```python
from build123d import *

# Parameters (mm, degrees)
SKETCH1_W                = 60
SKETCH1_H                = 60
BOSS_EXTRUDE1_DEPTH      = 41
M3_CLEARANCE_HOLE1_D     = 3.4
M3_CLEARANCE_HOLE1_DEPTH = 7
M3_CLEARANCE_HOLE1_TIP   = 1.021463052
SKETCH4_W                = 50
SKETCH4_H                = 50
BOSS_EXTRUDE2_DEPTH      = 28
SKETCH5_W                = 56
SKETCH5_H                = 56
BOSS_EXTRUDE3_DEPTH      = 18


with BuildPart() as part:
    # Sketch1 → Boss-Extrude1 (new body)
    with BuildSketch(Plane(origin=(0, 0, 0), x_dir=(1, 0, 0), z_dir=(0, 1, 0))):
        with Locations((30, 30)):
            Rectangle(SKETCH1_W, SKETCH1_H)
    extrude(amount=BOSS_EXTRUDE1_DEPTH)

    # M3 Clearance Hole1
    with Locations(Plane(origin=(0, 0, 0), x_dir=(-1, 0, 0), z_dir=(0, -1, 0))):
        with Locations((-3.5, 3.5), (-56.5, 3.5), (-56.5, 56.5), (-3.5, 56.5)):
            Hole(M3_CLEARANCE_HOLE1_D / 2, depth=M3_CLEARANCE_HOLE1_DEPTH)
            with Locations((0, 0, -(M3_CLEARANCE_HOLE1_DEPTH + M3_CLEARANCE_HOLE1_TIP / 2))):  # 118° drill point
                Cone(0, M3_CLEARANCE_HOLE1_D / 2, M3_CLEARANCE_HOLE1_TIP, mode=Mode.SUBTRACT)

    # Sketch4 → Boss-Extrude2 (add)
    with BuildSketch(Plane(origin=(0, 41, 0), x_dir=(1, 0, 0), z_dir=(0, 1, 0))):
        with Locations((30, 30)):
            Rectangle(SKETCH4_W, SKETCH4_H)
    extrude(amount=BOSS_EXTRUDE2_DEPTH)

    # Sketch5 → Boss-Extrude3 (add)
    with BuildSketch(Plane(origin=(0, 69, 0), x_dir=(1, 0, 0), z_dir=(0, 1, 0))):
        with Locations((30, 30)):
            Rectangle(SKETCH5_W, SKETCH5_H)
    extrude(amount=BOSS_EXTRUDE3_DEPTH)


solid = part.part
```
The listing builds one solid part. Answer for the finished solid, in the listing's coordinates (mm). A direction names the side the tool comes from. Coordinates: 2 decimals unless noted, no trailing zeros. Write each loop counter-clockwise with the first axis right and the second up, starting at its lowest first coordinate (ties: lowest second). Pieces come first, ordered by that corner, then holes. Notation, with made-up numbers: M 68.5,-23.5 L 83.5,-23.5 A4 cw 83.5,-16.5 Z; hole C 66,41 d9. An arc over 180 degrees is marked long. Use a Markdown table: item, result. Add a question column.
1. For a pull along Y with two mould halves and no side action, classify faces 1 (the flat face through (55, 55, -30)), 2 (the flat face through (30, 87, -30)), 3 (the flat face through (30, 20, -60)) as +Y half, -Y half, draft (parallel to the pull), parting line (faces both ways), or undercut.
2. Section B-B (z = -22) is taken. Give the vertices of the cut face in (x, y).
3. Section A-A (x = 10) is taken. Give the vertices of the cut face in (y, z), plus the area to 3 significant figures.
4. Given P1, Ø20, axis at x = 28, y = 81.5, coming from the +Z side; P2, Ø6, axis at x = 26.5, y = 65.5, coming from the +Z side; P3, Ø22.5, axis at y = 57, z = -25.5, coming from the +X side, each flat-ended and moving along its own axis, determine where each tip first touches the part or whether it passes through.
5. Section C-C (y = 56) is taken. Give the vertices of the cut face in (x, z).
6. Which of the six approach directions +Z, -Z, +X, -X, +Y, -Y give full straight-line access (tool end or side, diameter ignored) to faces 4 (the flat face through (30, 78, -2)), 5 (the flat face through (2, 78, -30)), 6 (the flat face through (56, 41, -30)), 7 (the cylindrical face through (54.8, 3.55, -3.57))?
7. Straight lines are drawn through the part: line 1 along X through (y, z) = (5, -56.5); line 2 along Z through (x, y) = (56.5, 5.5); line 3 along Y through (x, z) = (56, -14). For each, find the intervals that lie inside material, in ascending order. Write a range as [from, to].
Data:
| question | item | result |
|---|---|---|
| 1 | face 1 | undercut |
| 1 | face 2 | +Y half |
| 1 | face 3 | draft |
| 2 | outline | M 0,0 L 60,0 L 60,41 L 55,41 L 55,69 L 58,69 L 58,87 L 2,87 L 2,69 L 5,69 L 5,41 L 0,41 Z |
| 3 | outline | M 0,-60 L 41,-60 L 41,-55 L 69,-55 L 69,-58 L 87,-58 L 87,-2 L 69,-2 L 69,-5 L 41,-5 L 41,0 L 0,0 Z |
| 3 | area | 4,870 mm2 |
| 4 | P1 | stops at z = -2 |
| 4 | P2 | stops at z = -5 |
| 4 | P3 | stops at x = 55 |
| 5 | outline | M 5,-55 L 55,-55 L 55,-5 L 5,-5 Z |
| 6 | face 4 | +Z, +X, -X, +Y |
| 6 | face 5 | +Z, -Z, -X, +Y |
| 6 | face 6 | none |
| 6 | face 7 | -Y |
| 7 | line 1 | x = [0, 1.8], [5.2, 54.8], [58.2, 60] |
| 7 | line 2 | z = [-60, -58.2], [-54.8, -5.2], [-1.8, 0] |
| 7 | line 3 | y = [0, 41], [69, 87] |
